Autodesk Fusion 360 part; units mm, degrees
sketch "Sketch1" plane through (0, 0, 0) normal (0, 1, 0) x (1, 0, 0)
  line L0 (-60.0453, 0.0038) -> (60.0453, 0.0038)
  line L1 (60.0453, 0.0038) -> (60.0453, -10.0038)
  line L2 (60.0453, -10.0038) -> (-60.0453, -10.0038)
  line L3 (-60.0453, -10.0038) -> (-60.0453, 0.0038)
  line L4 (-60.0453, 0.0038) -> (60.0453, -10.0038) construction
  line L5 (60.0453, 0.0038) -> (-60.0453, -10.0038) construction
  line L6 (-30, -10) -> (30, -10)
  line L7 (30, -10) -> (30, -30)
  line L8 (-30, -30) -> (-30, -10)
  line L9 (-30, -10) -> (30, -30) construction
  line L10 (30, -10) -> (-30, -30) construction
  arc A0 (-30, -30) -> (30, -30) centre (0, -30) ccw
  circle A1 centre (0, -30) radius 15
  line L11 (30, -30) -> (15, -30)
  line L12 (-15, -30) -> (-30, -30)
  point P0 (0, -5)
  point P1 (0, -20)
  dimension "d3" = 60
  dimension "d4" = 20
sketch "Sketch2" plane through (0, 0, 0) normal (0, 1, 0) x (1, 0, 0)
  line L0 (60, 30) -> (-60, 30)
  line L1 (-60, 30) -> (-60, 20)
  line L2 (-60, 20) -> (-30, 20)
  line L3 (-30, 20) -> (-30, 0)
  arc A0 (-30, 0) -> (30, 0) centre (0, 0) ccw
  line L4 (30, 0) -> (30, 20)
  line L5 (30, 20) -> (60, 20)
  line L6 (60, 20) -> (60, 30)
  dimension "d11" = 120
  dimension "d12" = 60
  dimension "d13" = 30
  dimension "d14" = 30
  dimension "d15" = 10
extrude "Extrude2" add sketch "Sketch2" along normal blind 30
sketch "Sketch3" plane through (0, 0, 0) normal (0, -1, 0) x (1, 0, 0)
  line L0 (60, -30) -> (60, -20)
  line L1 (60, -20) -> (30, -20)
  line L2 (30, -20) -> (30, 0)
  arc A0 (30, 0) -> (-30, 0) centre (0, 0) ccw
  line L3 (-30, 0) -> (-30, -20)
  line L4 (-30, -20) -> (-60, -20)
  line L5 (-60, -20) -> (-60, -30)
  line L6 (-60, -30) -> (60, -30)
  circle A1 centre (0, 0) radius 15
  dimension "d18" = 30
extrude "Extrude3" cut sketch "Sketch3" against normal blind 30 contours A1
fillet "Fillet5" radius 4 2 edges at (-30, 15, -20) (30, 15, -20)
Part model, mm, in its own coordinate system. A direction names the side the tool comes from. Round coordinates to 2 decimals unless told otherwise and drop trailing zeros. Loops run counter-clockwise (first coordinate to the right, second up) from the corner with the lowest first, then second, coordinate; pieces in that order, holes last. Notation, with made-up numbers: (62.25, 81.5) -> (114.25, 81.5) arc R24 ccw to (114.25, 104.5) -> close; hole circle Ø4 at (62.5, 18). An arc over 180 degrees is marked (long way). Use one line per item in the form item = value. Start each with the question number.
Item 1: Drill centre lines: line 1 along Z through (x, y) = (0, 11.25); line 2 along Z through (x, y) = (-47, 20.25); line 3 along X through (y, z) = (5.25, 3). Where is each one in solid material? Low to high.
Item 2: Band-saw the part on D-D (x = 38). List the corners of the cut face in (y, z).
Item 3: Band-saw the part on C-C (z = 9). List the corners of the cut face in (x, y).
Item 4: Two-plate mould, pull along Z, no slides. Class faces 1 (the flat face through (30, 15, -8)), 2 (the cylindrical face through (-14.985, 14.79, 0.66)), 3 (the cylindrical face through (-31.141, 15.21, -18.797)): released by +Z, released by -Z, zero draft, split by the parting line, or undercut.
Item 5: Band-saw the part on A-A (x = 0). List the corners of the cut face in (y, z), plus the area to 3 significant figures.
Item 6: Drop flat-ended pins along their axis: pin 1 Ø4 at (y, z) = (11, -12) entering from +X; pin 2 Ø4 at (x, y) = (-20, 19.5) entering from +Z; pin 3 Ø12 at (x, z) = (3, -6.5) entering from -Y; pin 4 Ø1.5 at (y, z) = (27, 8.5) entering from +X. Give the stop position or say it passes through.
Item 7: Band-saw the part on B-B (y = 26.25). List the corners of the cut face in (x, z), plus the area to 3 significant figures.
Item 8: Tool access for faces 4 (the flat face through (-1, 30, -20)), 5 (the flat face through (47, 15, -20)), 6 (the flat face through (-47, 15, -20)): list every direction of +Z, -Z, +X, -X, +Y, -Y with a clear straight run to the whole face (end or side of a thin tool).
Data:
q1.line_1 = -30 to -15, 15 to 30
q1.line_2 = -30 to -20
q1.line_3 = -29.85 to -14.7, 14.7 to 29.85
q2.outline = (0, -30) -> (30, -30) -> (30, -20) -> (0, -20) -> close
q3.outline = (-28.62, 0) -> (-12, 0) -> (-12, 30) -> (-28.62, 30) -> close; (12, 0) -> (28.62, 0) -> (28.62, 30) -> (12, 30) -> close
q4.face_1 = zero draft
q4.face_2 = undercut
q4.face_3 = released by +Z
q5.outline = (0, -30) -> (30, -30) -> (30, -15) -> (0, -15) -> close; (0, 15) -> (30, 15) -> (30, 30) -> (0, 30) -> close
q5.area = 900 mm^2
q6.pin_1 = 30
q6.pin_2 = 24
q6.pin_3 = through
q6.pin_4 = 28.98
q7.outline = (-60, -30) -> (60, -30) -> (60, -20) -> (34, -20) arc R4 cw to (30, -16) -> (30, 0) arc R30 ccw to (-30, 0) -> (-30, -16) arc R4 cw to (-34, -20) -> (-60, -20) -> close; hole circle Ø30 at (0, 0)
q7.area = 3,110 mm^2
q8.face_4 = +Z, -Z, +X, -X, +Y
q8.face_5 = +Z, +X, +Y, -Y
q8.face_6 = +Z, -X, +Y, -Y
